Geometry check sheet. Reference: the model listing, model coordinates, mm. Face numbers are marked on the shaded views. A direction names the side the tool comes from. Give positions to 0.01 mm unless a question says otherwise; leave off trailing zeros. Order: outer loops, then holes, each group sorted by start corner. A loop starts at its lowest first (then second) coordinate and runs counter-clockwise, first axis right, second up.
from build123d import *

# Parameters (mm, degrees)
SALIENTE_EXTRUIR1_DEPTH = 3
CROQUIS2_R              = 2.75
SALIENTE_EXTRUIR2_DEPTH = 8
CROQUIS3_R              = 2.25
SALIENTE_EXTRUIR3_DEPTH = 8
CORTAR_EXTRUIR1_DEPTH   = 10
CROQUIS5_R              = 2.5
CORTAR_EXTRUIR2_DEPTH   = 2


with BuildPart() as part:
    # Croquis1 → Saliente-Extruir1 (new body)
    with BuildSketch(Plane.XY):
        with BuildLine():
            Line((-13.118348224, -13.346885602), (-5.358962429, -8.729934305))
            ThreePointArc((-5.358962429, -8.729934305), (0, -10.243545836), (5.358962429, -8.729934305))
            Line((5.358962429, -8.729934305), (13.118348224, -13.346885602))
            ThreePointArc((13.118348224, -13.346885602), (19.97194541, -11.606711584), (18.231771393, -4.753114398))
            Line((18.231771393, -4.753114398), (10.243545836, 0))
            ThreePointArc((10.243545836, 0), (8.83594818, 5.182301714), (5, 8.94037087))
            Line((5, 8.94037087), (5, 18.2))
            ThreePointArc((5, 18.2), (0, 23.2), (-5, 18.2))
            Line((-5, 18.2), (-5, 8.94037087))
            ThreePointArc((-5, 8.94037087), (-8.83594818, 5.182301714), (-10.243545836, 0))
            Line((-10.243545836, 0), (-18.231771393, -4.753114398))
            ThreePointArc((-18.231771393, -4.753114398), (-19.97194541, -11.606711584), (-13.118348224, -13.346885602))
        make_face()
    extrude(amount=SALIENTE_EXTRUIR1_DEPTH)

    # Croquis2 → Saliente-Extruir2 (add)
    with BuildSketch(Plane.XY.offset(3)):
        with Locations((0, 18.2)):
            Circle(CROQUIS2_R)
        with Locations((15.675059808, -9.05)):
            Circle(CROQUIS2_R)
        with Locations((-15.675059808, -9.05)):
            Circle(CROQUIS2_R)
    extrude(amount=SALIENTE_EXTRUIR2_DEPTH)

    # Croquis3 → Saliente-Extruir3 (add)
    with BuildSketch(Plane.XY.offset(3)):
        Circle(CROQUIS3_R)
    extrude(amount=SALIENTE_EXTRUIR3_DEPTH)

    # Croquis4 → Cortar-Extruir1 (cut)
    with BuildSketch(Plane(origin=(0, 0, 0), x_dir=(-1, 0, 0), z_dir=(0, 0, -1))):
        with BuildLine():
            Line((-4, 2.5), (-4, 4))
            Line((-4, 4), (-2.5, 4))
            ThreePointArc((-2.5, 4), (-5.060660172, 5.060660172), (-4, 2.5))
        make_face()
        with BuildLine():
            Line((-2.5, 4), (-4, 4))
            Line((-4, 4), (-4, 2.5))
            ThreePointArc((-4, 2.5), (-2.939339828, 2.939339828), (-2.5, 4))
        make_face()
        with BuildLine():
            ThreePointArc((5.5, 4), (4, 5.5), (2.5, 4))
            Line((2.5, 4), (4, 4))
            Line((4, 4), (4, 2.5))
            ThreePointArc((4, 2.5), (5.060660172, 2.939339828), (5.5, 4))
        make_face()
        with BuildLine():
            Line((4, 4), (2.5, 4))
            ThreePointArc((2.5, 4), (2.939339828, 2.939339828), (4, 2.5))
            Line((4, 2.5), (4, 4))
        make_face()
        with BuildLine():
            ThreePointArc((5.5, -4), (5.060660172, -2.939339828), (4, -2.5))
            Line((4, -2.5), (4, -4))
            Line((4, -4), (2.5, -4))
            ThreePointArc((2.5, -4), (4, -5.5), (5.5, -4))
        make_face()
        with BuildLine():
            Line((4, -4), (4, -2.5))
            ThreePointArc((4, -2.5), (2.939339828, -2.939339828), (2.5, -4))
            Line((2.5, -4), (4, -4))
        make_face()
        with BuildLine():
            ThreePointArc((-2.5, -4), (-2.939339828, -2.939339828), (-4, -2.5))
            Line((-4, -2.5), (-4, -4))
            Line((-4, -4), (-2.5, -4))
        make_face()
        with BuildLine():
            Line((-4, -4), (-4, -2.5))
            ThreePointArc((-4, -2.5), (-5.060660172, -5.060660172), (-2.5, -4))
            Line((-2.5, -4), (-4, -4))
        make_face()
    extrude(amount=-CORTAR_EXTRUIR1_DEPTH, mode=Mode.SUBTRACT)

    # Croquis5 → Cortar-Extruir2 (cut)
    with BuildSketch(Plane.XY.offset(3)):
        with Locations((-4, 4)):
            Circle(CROQUIS5_R)
        with Locations((4, 4)):
            Circle(CROQUIS5_R)
        with Locations((4, -4)):
            Circle(CROQUIS5_R)
        with Locations((-4, -4)):
            Circle(CROQUIS5_R)
    extrude(amount=-CORTAR_EXTRUIR2_DEPTH, mode=Mode.SUBTRACT)


solid = part.part
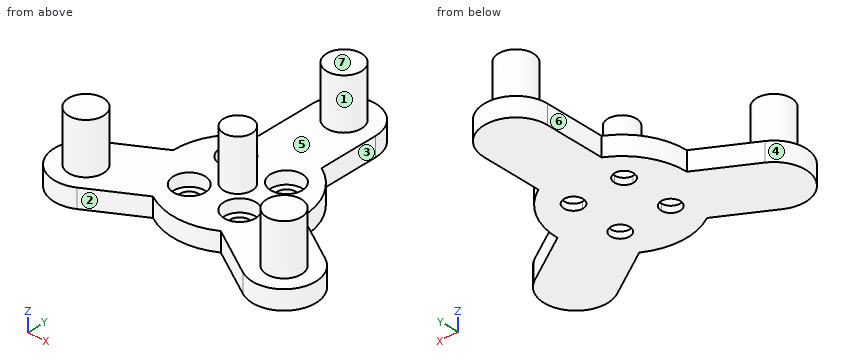
Item 1: Draft check along Y on the marked faces 1, 2, 3 and 4. Enter one of: released by +Y, released by -Y, zero draft, split by the parting line, or undercut.
Reported:
face 1: undercut
face 2: released by -Y
face 3: zero draft
face 4: split by the parting line
Item 2: Scan lines: L1, parallel to X at y = -4, z = 0.3; L2, parallel to Y at x = 4, z = 2.35; L3, parallel to Y at x = 4, z = 0.5. Record each from-to range of solid material in increasing order.
Reported:
L1: x = -16.97 to -5.5, -2.5 to 2.5, 5.5 to 16.97
L2: y = -9.43 to -6.5, -1.5 to 1.5, 6.5 to 21.2
L3: y = -9.43 to -5.5, -2.5 to 2.5, 5.5 to 21.2
Item 3: Sectioned sample at D-D (y = 11.5). Enter the section's corners in (x, z).
Reported:
outline: (-5, 0) - (5, 0) - (5, 3) - (-5, 3) - close
Item 4: Set-up check for the marked faces 5, 6 and 7: record each of +Z, -Z, +X, -X, +Y, -Y from which the full face is reachable in a straight line by a thin tool's end or side.
Reported:
face 5: +Z
face 6: +Z, -Z, -X, +Y
face 7: +Z, +X, -X, +Y, -Y
Item 5: Sectioned sample at C-C (x = -1). Enter the section's corners in (y, z), and give its area (3 significant figures).
Reported:
outline: (-10.19, 0) - (23.1, 0) - (23.1, 3) - (20.76, 3) - (20.76, 11) - (15.64, 11) - (15.64, 3) - (2.02, 3) - (2.02, 11) - (-2.02, 11) - (-2.02, 3) - (-10.19, 3) - close
area: 173 mm2
Item 6: Gauge pin test, flat ends, axial feed: pin 1 (2.5 mm diameter, centred on x = 3.5, y = -4.5, fed in from +Z); pin 2 (1.5 mm diameter, centred on y = 11.5, z = 2, fed in from -X); pin 3 (4 mm diameter, centred on x = -12, z = 8, fed in from -Y). Record the tip position at first contact, or that the pin passes through.
Reported:
pin 1: stops at z = 1
pin 2: stops at x = -5
pin 3: stops at y = -11.23
Item 7: Sectioned sample at B-B (x = 4.5). Enter the section's corners in (y, z), and give its area (3 significant figures).
Reported:
outline: (-9.2, 0) - (-5.41, 0) - (-5.41, 1) - (-6.45, 1) - (-6.45, 3) - (-9.2, 3) - close; (-2.59, 0) - (2.59, 0) - (2.59, 1) - (1.55, 1) - (1.55, 3) - (-1.55, 3) - (-1.55, 1) - (-2.59, 1) - close; (5.41, 0) - (20.38, 0) - (20.38, 3) - (6.45, 3) - (6.45, 1) - (5.41, 1) - close
area: 63.5 mm2
Item 8: Sectioned sample at A-A (z = 4.75). Enter the section's corners in (x, y).
Reported:
outline: circle Ø5.5 at (-15.68, -9.05); circle Ø5.5 at (0, 18.2); circle Ø4.5 at (0, 0); circle Ø5.5 at (15.68, -9.05)
